```python
from build123d import *

# Parameters (mm, degrees)
SKETCH1_R           = 10
BOSS_EXTRUDE2_DEPTH = 45
SKETCH4_OUTSIDE_W   = 32.63
SKETCH4_OUTSIDE_H   = 32.63
SKETCH4_OUTSIDE_W_2 = 13
SKETCH4_OUTSIDE_H_2 = 20
CUT_EXTRUDE2_DEPTH  = 15
FILLET2_R           = 3
BOSS_EXTRUDE3_START = -5
SKETCH7_W           = 2.5
SKETCH7_H           = 2.5
BOSS_EXTRUDE3_DEPTH = 5.078433
SKETCH8_W           = 5
SKETCH8_H           = 5
BOSS_EXTRUDE4_DEPTH = 2.5
BOSS_EXTRUDE6_START = -0.202041
SKETCH9_R           = 2
BOSS_EXTRUDE6_DEPTH = 2.202041
SKETCH10_R          = 3.5
BOSS_EXTRUDE7_DEPTH = 2
SKETCH11_W          = 6.400657923
SKETCH11_H          = 7.5
BOSS_EXTRUDE8_DEPTH = 2


with BuildPart() as part:
    # Sketch1 → Boss-Extrude2 (new body)
    with BuildSketch(Plane(origin=(0, 0, 0), x_dir=(1, 0, 0), z_dir=(0, 1, 0))):
        Circle(SKETCH1_R)
    extrude(amount=BOSS_EXTRUDE2_DEPTH)

    # Sketch4 outside → Cut-Extrude2 (cut)
    with BuildSketch(Plane(origin=(0, 45, 0), x_dir=(1, 0, 0), z_dir=(0, 1, 0))):
        Rectangle(SKETCH4_OUTSIDE_W, SKETCH4_OUTSIDE_H)
        Rectangle(SKETCH4_OUTSIDE_W_2, SKETCH4_OUTSIDE_H_2, mode=Mode.SUBTRACT)
    extrude(amount=-CUT_EXTRUDE2_DEPTH, mode=Mode.SUBTRACT)

    # Sketch5 → Cut-Revolve1 (revolve, cut)
    with BuildSketch(Plane.ZY.offset(6.5)):
        with BuildLine():
            Line((0, 42.792409201), (0, 37.792409201))
            ThreePointArc((0, 37.792409201), (-2.5, 40.292409201), (0, 42.792409201))
        make_face()
    cut_revolve1 = revolve(axis=Axis((-6.5, 42.792409201, 0), (0, -1, 0)), mode=Mode.SUBTRACT)

    # Mirror2: Cut-Revolve1 across plane
    add(cut_revolve1.mirror(Plane(origin=(0, 0, 0), x_dir=(0, 0, 1), z_dir=(1, 0, 0))), mode=Mode.SUBTRACT)

    # Fillet2
    fillet2_edges = [part.edges().sort_by_distance(p)[0] for p in [
        (-10, 0, 0),
    ]]
    fillet(fillet2_edges, radius=FILLET2_R)

    # Sketch7 → Boss-Extrude3 (add)
    with BuildSketch(Plane.XY.offset(-10).offset(BOSS_EXTRUDE3_START)):
        with Locations((0, 25)):
            Rectangle(SKETCH7_W, SKETCH7_H)
    extrude(amount=BOSS_EXTRUDE3_DEPTH)

    # Sketch8 → Boss-Extrude4 (add)
    with BuildSketch(Plane(origin=(0, 0, -15), x_dir=(-1, 0, 0), z_dir=(0, 0, -1))):
        with Locations((0, 25)):
            Rectangle(SKETCH8_W, SKETCH8_H)
    extrude(amount=BOSS_EXTRUDE4_DEPTH)

    # Sketch9 → Boss-Extrude6 (add)
    with BuildSketch(Plane.XY.offset(10).offset(BOSS_EXTRUDE6_START)):
        with Locations((0, 25)):
            Circle(SKETCH9_R)
    extrude(amount=BOSS_EXTRUDE6_DEPTH)

    # Sketch10 → Boss-Extrude7 (add)
    with BuildSketch(Plane.XY.offset(12)):
        with Locations((0, 24.995165492)):
            Circle(SKETCH10_R)
    extrude(amount=BOSS_EXTRUDE7_DEPTH)

    # Sketch11 → Boss-Extrude8 (add)
    with BuildSketch(Plane(origin=(6.5, 0, 0), x_dir=(0, 0, -1), z_dir=(1, 0, 0))):
        with Locations((10.799671038, 41.25)):
            Rectangle(SKETCH11_W, SKETCH11_H)
    boss_extrude8 = extrude(amount=-BOSS_EXTRUDE8_DEPTH)

    # Mirror3: Boss-Extrude8 across plane
    add(boss_extrude8.mirror(Plane(origin=(0, 0, 0), x_dir=(0, 0, 1), z_dir=(1, 0, 0))))


solid = part.part
```
The model under review builds one solid part; all positions refer to its coordinate system, in mm. A direction names the side the tool comes from. Round coordinates to 2 decimals unless told otherwise and drop trailing zeros. Order: outer loops, then holes, each group sorted by start corner. A loop starts at its lowest first (then second) coordinate and runs counter-clockwise, first axis right, second up.
Item 1: For pin 1 (3 mm diameter, centred on y = 25.5, z = -12, fed in from +X); pin 2 (10 mm diameter, centred on x = 4, y = 7.5, fed in from -Z); pin 3 (2 mm diameter, centred on x = -5, y = 35.5, fed in from +Z), all flat-tipped, find the tip position at first contact; note any pin that passes through.
Working result:
pin 1: stops at x = 1.25
pin 2: stops at z = -10
pin 3: stops at z = 9.17
Item 2: Add section D-D, the plane y = 31.5. State the section outline as (x, z) points, and give its area (3 significant figures).
Working result:
outline: (-6.5, -7.6) arc R10 ccw to (6.5, -7.6) - (6.5, 7.6) arc R10 ccw to (-6.5, 7.6) - close
area: 240 mm2
Item 3: Draft analysis for pull direction Z (two halves, no side actions). For faces 4 (the flat face through (0, 25, -17.5)), 5 (the flat face through (1.25, 25, -12)), 6 (the flat face through (0, 0, 0)), state which applies: released by +Z, released by -Z, zero draft, split by the parting line, or undercut.
Working result:
face 4: released by -Z
face 5: undercut
face 6: zero draft
Item 4: Add section A-A, the plane z = 0. State the section outline as (x, y) points.
Working result:
outline: (-10, 3) arc R3 ccw to (-7, 0) - (7, 0) arc R3 ccw to (10, 3) - (10, 30) - (6.5, 30) - (6.5, 37.79) arc R2.5 cw to (6.5, 42.79) - (6.5, 45) - (-6.5, 45) - (-6.5, 42.79) arc R2.5 cw to (-6.5, 37.79) - (-6.5, 30) - (-10, 30) - close
Item 5: Machinability: for faces 1 (the flat face through (6.5, 38, -3)), 2 (the flat face through (0, 27.5, -16)), 3 (the flat face through (6, 37.5, -11)), which of the approach directions +Z, -Z, +X, -X, +Y, -Y give a long, thin tool a straight path to every point of the face, cutting with its end or side? Answer none if there is none.
Working result:
face 1: +Z, -Z, +X, +Y
face 2: -Z, +X, -X, +Y
face 3: -Z, +X, -Y
Item 6: Add section B-B, the plane x = 0. State the section outline as (y, z) points, and give its area (3 significant figures).
Working result:
outline: (0, -7) arc R3 ccw to (3, -10) - (23.75, -10) - (23.75, -15) - (22.5, -15) - (22.5, -17.5) - (27.5, -17.5) - (27.5, -15) - (26.25, -15) - (26.25, -10) - (45, -10) - (45, 10) - (27, 10) - (27, 12) - (28.5, 12) - (28.5, 14) - (21.5, 14) - (21.5, 12) - (23, 12) - (23, 10) - (3, 10) arc R3 ccw to (0, 7) - close
area: 943 mm2
Item 7: To check wall thickness, follow probe 1 along Y at (x, z) = (-6.25, -8); probe 2 along X at (y, z) = (42, -11.5); probe 3 along X at (y, z) = (40, -6). State the ranges of each line that lie inside material, in increasing order.
Working result:
probe 1: y = 37.5 to 45
probe 2: x = -6.5 to -4.5, 4.5 to 6.5
probe 3: x = -6.5 to 6.5
Item 8: Add section C-C, the plane y = 20. State the section outline as (x, z) points, and give its area (3 significant figures).
Working result:
outline: circle Ø20 at (0, 0)
area: 314 mm2
